```python
from build123d import *

# Parameters (mm, degrees)
F0_W      = 337.0173126459
F0_H      = 86.0028490424
F1_DEPTH  = 7.62
F2_W      = 3.4302696586
F2_H      = 86.0028490424
F3_DEPTH  = 279.4
F4_W      = 86.0028490424
F4_H      = 4.4084019136
F5_DEPTH  = 108.712
F6_W      = 43.0014245212
F6_H      = 4.1845664382
F7_DEPTH  = 108.712
F8_W      = 86.0028490424
F8_H      = 5.0613901806
F9_DEPTH  = 108.712
F10_W     = 2.5949749823
F10_H     = 86.0028490424
F11_DEPTH = 282.702
F12_W     = 84.5208009705
F12_H     = 86.0028490424
F13_DEPTH = 25.4
F14_W     = 2.429779619
F14_H     = 86.0028490424
F15_DEPTH = 279.4
F16_W     = 86.0028490424
F16_H     = 5.0492010307
F17_DEPTH = 84.836
F18_W     = 86.0028490424
F18_H     = 2.9006898403
F19_DEPTH = 84.836
F20_W     = 86.0028490424
F20_H     = 3.3634305
F21_DEPTH = 85.09
F22_W     = 86.0028490424
F22_H     = 2.3629367352
F23_DEPTH = 85.09
F24_W     = 86.0028490424
F24_H     = 3.8478970528
F25_DEPTH = 85.09
F26_W     = 86.0028490424
F26_H     = 3.7884193933
F27_DEPTH = 85.09
F29_W     = 137.556899339
F29_H     = 86.3062888384
F30_DEPTH = 25.4
F31_W     = 86.0028490424
F31_H     = 1.7304397297
F32_DEPTH = 143.256
F33_W     = 86.0028490424
F33_H     = 5.6310913754
F34_DEPTH = 143.256
F35_W     = 2.9041429413
F35_H     = 86.0028490424
F36_DEPTH = 300.5836
F37_W     = 86.0028490424
F37_H     = 3.6729436779
F38_DEPTH = 141.732
F39_W     = 109.4675436616
F39_H     = 2.797678113
F40_DEPTH = 17.78
F41_W     = 2.5949749823
F41_H     = 2.8018429875
F42_DEPTH = 17.0688
F43_DEPTH = 83.1596
F44_W     = 109.4675436616
F44_H     = 1.4792491037
F45_DEPTH = 83.058
F46_DEPTH = 177.8
F47_W     = 2.9938668013
F47_H     = 86.0028490424
F48_DEPTH = 177.8
F49_W     = 2.7467114851
F49_H     = 86.0028490424
F50_DEPTH = 177.8
F51_DEPTH = 17.78
F52_W     = 2.9041429413
F52_H     = 86.0028490424
F53_DEPTH = 177.8
F54_W     = 86.0028490424
F54_H     = 21.5720179844
F55_DEPTH = 226.06


with BuildPart() as f1:
    # F0 (on Top) → F1 (new body)
    with BuildSketch(Plane.XY):
        with Locations((-12.588955462, 43.0014245212)):
            Rectangle(F0_W, F0_H)
    extrude(amount=F1_DEPTH)

    # F2 (on face) → F3 (join)
    with BuildSketch(Plane.XY.offset(7.62)):
        with Locations((-73.3452029526, 43.0014245212)):
            Rectangle(F2_W, F2_H)
    extrude(amount=F3_DEPTH)

    # F4 (on face) → F5 (join)
    with BuildSketch(Plane(origin=(-75.0603377819, 0, 0), x_dir=(0, -1, 0), z_dir=(-1, 0, 0))):
        with Locations((-43.0014245212, 145.1157990432)):
            Rectangle(F4_W, F4_H)
    extrude(amount=F5_DEPTH)

    # F6 (on face) → F7 (join)
    with BuildSketch(Plane(origin=(-75.0603377819, 0, 0), x_dir=(0, -1, 0), z_dir=(-1, 0, 0))):
        with Locations((-64.5021367818, 120.2528215945)):
            Rectangle(F6_W, F6_H)
    extrude(amount=F7_DEPTH)

    # F8 (on face) → F9 (join)
    with BuildSketch(Plane(origin=(-75.0603377819, 0, 0), x_dir=(0, -1, 0), z_dir=(-1, 0, 0))):
        with Locations((-43.0014245212, 284.4893049097)):
            Rectangle(F8_W, F8_H)
    extrude(amount=F9_DEPTH)

    # F10 (on face) → F11 (join)
    with BuildSketch(Plane(origin=(0, 0, 281.9586098194), x_dir=(1, 0, 0), z_dir=(0, 0, -1))):
        with Locations((-182.4748502908, -43.0014245212)):
            Rectangle(F10_W, F10_H)
    extrude(amount=F11_DEPTH)

    # F12 (on face) → F13 (join)
    with BuildSketch(Plane.XY.offset(7.62)):
        with Locations((-29.3696676381, 43.0014245212)):
            Rectangle(F12_W, F12_H)
    extrude(amount=-F13_DEPTH)

    # F14 (on face) → F15 (join)
    with BuildSketch(Plane.XY.offset(7.62)):
        with Locations((13.6984353885, 43.0014245212)):
            Rectangle(F14_W, F14_H)
    extrude(amount=F15_DEPTH)

    # F16 (on face) → F17 (join)
    with BuildSketch(Plane.YZ.offset(-71.6300681233)):
        with Locations((43.0014245212, 284.4953994846)):
            Rectangle(F16_W, F16_H)
    extrude(amount=F17_DEPTH)

    # F18 (on face) → F19 (join)
    with BuildSketch(Plane.YZ.offset(-71.6300681233)):
        with Locations((43.0014245212, 165.8845096827)):
            Rectangle(F18_W, F18_H)
    extrude(amount=F19_DEPTH)

    # F20 (on face) → F21 (join)
    with BuildSketch(Plane.YZ.offset(-71.6300681233)):
        with Locations((43.0014245212, 222.971111536)):
            Rectangle(F20_W, F20_H)
    extrude(amount=F21_DEPTH)

    # F22 (on face) → F23 (join)
    with BuildSketch(Plane.YZ.offset(-71.6300681233)):
        with Locations((43.0014245212, 133.7857097387)):
            Rectangle(F22_W, F22_H)
    extrude(amount=F23_DEPTH)

    # F24 (on face) → F25 (join)
    with BuildSketch(Plane.YZ.offset(-71.6300681233)):
        with Locations((43.0014245212, 92.8397625685)):
            Rectangle(F24_W, F24_H)
    extrude(amount=F25_DEPTH)

    # F26 (on face) → F27 (join)
    with BuildSketch(Plane.YZ.offset(-71.6300681233)):
        with Locations((43.0014245212, 47.3736973244)):
            Rectangle(F26_W, F26_H)
    extrude(amount=F27_DEPTH)

    # F29 (on face) → F30 (join)
    with BuildSketch(Plane.XY.offset(7.62)):
        with Locations((84.4397153705, 43.1531444192)):
            Rectangle(F29_W, F29_H)
    extrude(amount=-F30_DEPTH)

    # F31 (on face) → F32 (join)
    with BuildSketch(Plane.YZ.offset(14.913325198)):
        with Locations((43.0014245212, 146.4547801352)):
            Rectangle(F31_W, F31_H)
    extrude(amount=F32_DEPTH)

    # F33 (on face) → F34 (join)
    with BuildSketch(Plane.YZ.offset(14.913325198)):
        with Locations((43.0014245212, 284.2044543123)):
            Rectangle(F33_W, F33_H)
    extrude(amount=F34_DEPTH)

    # F35 (on face) → F36 (join)
    with BuildSketch(Plane(origin=(0, 0, 281.3889086246), x_dir=(1, 0, 0), z_dir=(0, 0, -1))):
        with Locations((156.7172537273, -43.0014245212)):
            Rectangle(F35_W, F35_H)
    extrude(amount=F36_DEPTH)

    # F37 (on face) → F38 (join)
    with BuildSketch(Plane.YZ.offset(14.913325198)):
        with Locations((43.0014245212, 216.1909261513)):
            Rectangle(F37_W, F37_H)
    extrude(amount=F38_DEPTH)

    # F39 (on face) → F40 (join)
    with BuildSketch(Plane(origin=(0, 0, 0), x_dir=(1, 0, 0), z_dir=(0, 0, -1))):
        with Locations((-126.3638399541, -84.6040099859)):
            Rectangle(F39_W, F39_H)
    extrude(amount=F40_DEPTH)

    # F41 (on face) → F42 (join)
    with BuildSketch(Plane(origin=(0, 0, -0.7433901806), x_dir=(1, 0, 0), z_dir=(0, 0, -1))):
        with Locations((-182.4748502908, -84.6019275486)):
            Rectangle(F41_W, F41_H)
    extrude(amount=F42_DEPTH)

    # F43 (add): a face of the model
    f43_faces = [f1.faces().sort_by_distance(p)[0] for p in [
        (-182.4748502908, 83.2010060549, -9.2777901806),
    ]]
    extrude(f43_faces, amount=F43_DEPTH)

    # F44 (on face) → F45 (join)
    with BuildSketch(Plane.XZ.offset(-83.2051709294)):
        with Locations((-126.3638399541, -17.0403754482)):
            Rectangle(F44_W, F44_H)
    extrude(amount=F45_DEPTH)

    # F46 (add): a face of the model
    f46_faces = [f1.faces().sort_by_distance(p)[0] for p in [
        (-182.4748502908, 43.0221275486, -17.8121901806),
    ]]
    extrude(f46_faces, amount=F46_DEPTH)

    # F47 (on face) → F48 (join)
    with BuildSketch(Plane(origin=(0, 0, -17.78), x_dir=(1, 0, 0), z_dir=(0, 0, -1))):
        with Locations((-70.1331347227, -43.0014245212)):
            Rectangle(F47_W, F47_H)
    extrude(amount=F48_DEPTH)

    # F49 (on face) → F50 (join)
    with BuildSketch(Plane(origin=(0, 0, -17.78), x_dir=(1, 0, 0), z_dir=(0, 0, -1))):
        with Locations((11.5173771046, -43.0014245212)):
            Rectangle(F49_W, F49_H)
    extrude(amount=F50_DEPTH)

    # F51 (add): a face of the model
    f51_faces = [f1.faces().sort_by_distance(p)[0] for p in [
        (154.2416736484, 43.0014245212, 0),
    ]]
    extrude(f51_faces, amount=F51_DEPTH)

    # F52 (on face) → F53 (join)
    with BuildSketch(Plane(origin=(0, 0, -19.1946913754), x_dir=(1, 0, 0), z_dir=(0, 0, -1))):
        with Locations((156.7172537273, -43.0014245212)):
            Rectangle(F52_W, F52_H)
    extrude(amount=F53_DEPTH)

    # F54 (on face) → F55 (join)
    with BuildSketch(Plane.YZ.offset(-68.6362013221)):
        with Locations((43.0014245212, -184.7939910078)):
            Rectangle(F54_W, F54_H)
    extrude(amount=F55_DEPTH)


solid = f1.part
```
Can you work these out from the model? Positions are in its coordinate system, mm. Give positions to 0.01 mm unless a question says otherwise; leave off trailing zeros. Loops run counter-clockwise (first coordinate to the right, second up) from the corner with the lowest first, then second, coordinate; pieces in that order, holes last. Notation, with made-up numbers: M -23,-2 L 24,-2 A29 ccw 24,18 Z; hole C 31,42 d4. An arc over 180 degrees is marked long. One line per question, with ' | ' between items. Start each with the question number.
Q1. If I drill on line 1 (Z direction, x = -128, y = 4.5); line 2 (X direction, y = 66, z = -146); line 3 (X direction, y = 74, z = 98.5), over which ranges is the centre line in solid material (lowest first)? Write a range as from..to.
Q2. If we section it at C-C (x = -19.5): State how many separate pieces and enclosed holes the cut face has, plus the area to 3 significant figures.
Q3. If we mould it in two halves opening along X, with no side actions, what happens to faces 1 (the flat face through (-14, 86.003, -10)), 2 (the flat face through (12.484, 42, 113)), 3 (the flat face through (158.169, 44, 48))? For each: +X half, -X half, draft (parallel to the pull), parting line (faces both ways), or undercut.
Q4. If we section it at A-A (x = -152): Please give me the cut outline in (y, z), plus the area to 3 significant figures.
Q5. If we section it at D-D (z = 158): Please give me the cut outline in (x, y), plus the area to 3 significant figures.
Q6. If we section it at B-B (z = -139.5): Please give me the cut outline in (x, y), plus the area to 3 significant figures.
Q7. For pin 1 Ø5 at (x, z) = (-141.5, -12) entering from -Y; pin 2 Ø10 at (x, y) = (101, 32) entering from -Z; pin 3 Ø12 at (x, z) = (0, -82.5) entering from +Y; pin 4 Ø4 at (x, y) = (-122.5, 76) entering from -Z, each with a flat end and sliding along its axis, tell me the tip position at first contact or that it passes through.
Computed:
1) line 1: z = -17.78..-16.3, 0..7.62, 142.91..147.32, 281.96..287.02 | line 2: x = -183.77..-181.18, -71.63..-68.64, 10.14..12.89, 155.27..158.17 | line 3: x = -183.77..-181.18, -75.06..-71.63, 12.48..14.91, 155.27..158.17
2) separate pieces: 8 | enclosed holes: 0 | area: 5,870 mm²
3) face 1: draft | face 2: undercut | face 3: +X half
4) outline: M 0,0 L 83.21,0 L 83.21,-16.3 L 0.15,-16.3 L 0.15,-17.78 L 86,-17.78 L 86,7.62 L 0,7.62 Z; M 0,142.91 L 86,142.91 L 86,147.32 L 0,147.32 Z; M 0,281.96 L 86,281.96 L 86,287.02 L 0,287.02 Z; M 43,118.16 L 86,118.16 L 86,122.35 L 43,122.35 Z | area: 1,820 mm²
5) outline: M -183.77,0 L -181.18,0 L -181.18,86 L -183.77,86 Z; M -75.06,0 L -71.63,0 L -71.63,86 L -75.06,86 Z; M 12.48,0 L 14.91,0 L 14.91,86 L 12.48,86 Z; M 155.27,0 L 158.17,0 L 158.17,86 L 155.27,86 Z | area: 977 mm²
6) outline: M -183.77,0.04 L -181.18,0.04 L -181.18,86 L -183.77,86 Z; M -71.63,0 L -68.64,0 L -68.64,86 L -71.63,86 Z; M 10.14,0 L 12.89,0 L 12.89,86 L 10.14,86 Z; M 155.27,0 L 158.17,0 L 158.17,86 L 155.27,86 Z | area: 967 mm²
7) pin 1: stops at y = 83.21 | pin 2: stops at z = -195.58 | pin 3: passes through | pin 4: stops at z = -17.78
